Can you work these out from the model? Positions are in its coordinate system, mm. Face numbers are marked on the shaded views. A direction names the side the tool comes from. Give positions to 0.01 mm unless a question says otherwise; leave off trailing zeros. Order: outer loops, then holes, each group sorted by start corner. A loop starts at its lowest first (then second) coordinate and runs counter-clockwise, first axis right, second up. Notation, with made-up numbers: M 21,27 L 78,27 A24 cw 78,48 Z; hole C -5,59.5 d9. An arc over 180 degrees is marked long. Answer as a JSON object with one key per item and string values.
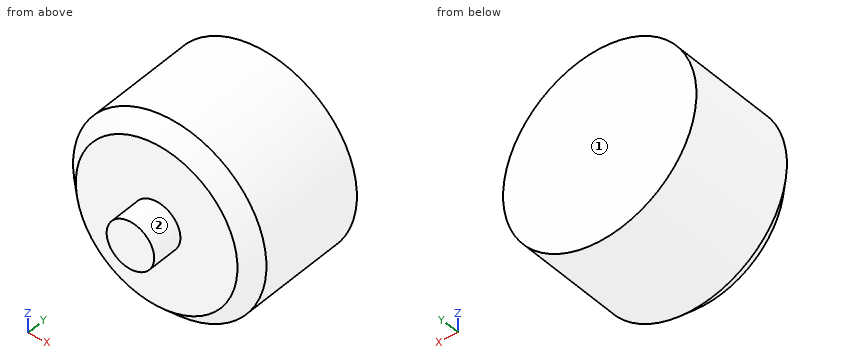
```python
from build123d import *

# Parameters (mm, degrees)
SKETCH_1_R      = 12.2
EXTRUDE_1_DEPTH = 15.8
CHAMFER_1_SIZE  = 2
SKETCH_2_R      = 3
EXTRUDE_2_DEPTH = 4


with BuildPart() as part:
    # 草图1 → 凸台-拉伸1 (new body)
    with BuildSketch(Plane(origin=(0, 0, 0), x_dir=(1, 0, 0), z_dir=(0, 1, 0))):
        with Locations(Location((0, 0, 0), (0, 0, 270))):
            Circle(SKETCH_1_R)
    extrude(amount=EXTRUDE_1_DEPTH)

    # 倒角1
    chamfer_1_edges = [part.edges().sort_by_distance(p)[0] for p in [
        (0, 0, -12.2),
    ]]
    chamfer(chamfer_1_edges, length=CHAMFER_1_SIZE)

    # 草图2 → 凸台-拉伸2 (add)
    with BuildSketch(Plane.XZ):
        with Locations(Location((0, 0, 0), (0, 0, 90))):
            Circle(SKETCH_2_R)
    extrude(amount=EXTRUDE_2_DEPTH)


solid = part.part
```
1) I want a section at A-A on z = 0. Write out the boundary of the cut face in (x, y).
Results found:
{"outline": "M -12.2,2 L -10.2,0 L -3,0 L -3,-4 L 3,-4 L 3,0 L 10.2,0 L 12.2,2 L 12.2,15.8 L -12.2,15.8 Z"}
2) I'm going to push flat-ended pins straight in: pin 1 Ø4 at (x, y) = (6, 6.5) entering from -Z; pin 2 Ø3 at (y, z) = (1.5, -6) entering from -X; pin 3 Ø10 at (y, z) = (8.5, -8.5) entering from +X. Where does each tip first touch, or does it pass through?
Results found:
{"pin 1": "stops at z = -11.53", "pin 2": "stops at x = -11.31", "pin 3": "stops at x = 11.69"}
3) I need wall thicknesses on L1, parallel to Y at x = -7, z = 0.5; L2, parallel to Z at x = 11.25, y = 7.5; L3, parallel to Z at x = -9, y = 0.5. Which ranges of each line are inside material? Lowest first, please.
Results found:
{"L1": "y = 0 to 15.8", "L2": "z = -4.72 to 4.72", "L3": "z = -5.79 to 5.79"}
4) I want a section at D-D on y = -1. Write out the boundary of the cut face in (x, z), and give its area (3 significant figures).
Results found:
{"outline": "C 0,0 d6", "area": "28.3 mm²"}
5) I want a section at B-B on x = 0. Write out the boundary of the cut face in (y, z).
Results found:
{"outline": "M -4,-3 L 0,-3 L 0,-10.2 L 2,-12.2 L 15.8,-12.2 L 15.8,12.2 L 2,12.2 L 0,10.2 L 0,3 L -4,3 Z"}
6) I want a section at C-C on y = 14.5. Write out the boundary of the cut face in (x, z), and give its area (3 significant figures).
Results found:
{"outline": "C 0,0 d24.4", "area": "468 mm²"}
7) For the marked faces 1 and 2, which set-ups out of +Z, -Z, +X, -X, +Y, -Y let a thin tool reach every point of the face, with its end or its side?
Results found:
{"face 1": "+Z, -Z, +X, -X, +Y", "face 2": "-Y"}
